Could you check a few things on this model? Use its own coordinates, in mm. Face numbers are marked on the shaded views. A direction names the side the tool comes from. Round coordinates to 2 decimals unless told otherwise and drop trailing zeros. Loops run counter-clockwise (first coordinate to the right, second up) from the corner with the lowest first, then second, coordinate; pieces in that order, holes last. Notation, with made-up numbers: M -2.5,30.5 L 52.5,30.5 A21 cw 52.5,37.5 Z; hole C 86.25,76 d8. An arc over 180 degrees is marked long. Answer in a Markdown table with one row per item.
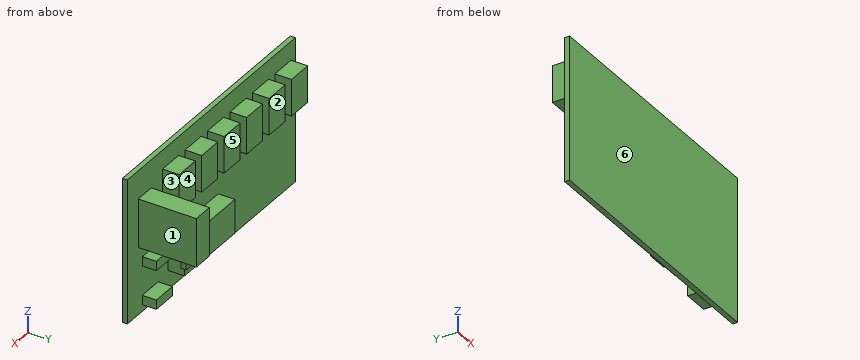
Autodesk Inventor part; units mm, degrees
ref_plane "YZ Plane" through (0, 0, 0) normal (1, 0, 0) x (0, 1, 0)
ref_plane "XZ Plane" through (0, 0, 0) normal (0, 1, 0) x (-1, 0, 0)
ref_plane "XY Plane" through (0, 0, 0) normal (0, 0, 1) x (1, 0, 0)
sketch "Sketch1" plane through (0, 0, 0) normal (0, 1, 0) x (-1, 0, 0)
  line L0 (-80, -43.475) -> (80, -43.475)
  line L1 (80, -43.475) -> (80, 43.475)
  line L2 (80, 43.475) -> (-80, 43.475)
  line L3 (-80, 43.475) -> (-80, -43.475)
  line L4 (-80, -43.475) -> (80, 43.475) construction
  line L5 (80, -43.475) -> (-80, 43.475) construction
  point P0 (0, 0)
  dimension "d0" = 160
  dimension "d1" = 86.95
extrude "Extrusion1" add sketch "Sketch1" along normal blind 3
sketch "Sketch2" plane through (0, 3, 0) normal (0, 1, 0) x (1, 0, 0)
  line L0 (-6.6, 31.775) -> (41.4, 31.775)
  line L1 (41.4, 31.775) -> (41.4, 11.375)
  line L2 (41.4, 11.375) -> (-6.6, 11.375)
  line L3 (-6.6, 11.375) -> (-6.6, 31.775)
  line L4 (80, -43.475) -> (80, 43.475)
  line L5 (-80, -43.475) -> (80, -43.475)
  line L6 (-75.9, -32.075) -> (-60.6, -32.075)
  line L7 (-60.6, -32.075) -> (-60.6, -9.975)
  line L8 (-60.6, -9.975) -> (-75.9, -9.975)
  line L9 (-75.9, -9.975) -> (-75.9, -32.075)
  line L10 (-80, 43.475) -> (-80, -43.475)
  line L11 (-54.5, -32.075) -> (-39.2, -32.075)
  line L12 (-39.2, -32.075) -> (-39.2, -9.975)
  line L13 (-39.2, -9.975) -> (-54.5, -9.975)
  line L14 (-54.5, -9.975) -> (-54.5, -32.075)
  line L15 (-33.1, -32.075) -> (-17.8, -32.075)
  line L16 (-17.8, -32.075) -> (-17.8, -9.975)
  line L17 (-17.8, -9.975) -> (-33.1, -9.975)
  line L18 (-33.1, -9.975) -> (-33.1, -32.075)
  line L19 (57.2, 2.825) -> (69.6, 2.825)
  line L20 (69.6, 2.825) -> (69.6, -26.475)
  line L21 (69.6, -26.475) -> (57.2, -26.475)
  line L22 (57.2, -26.475) -> (57.2, 2.825)
  line L23 (-11.7, -9.975) -> (-11.7, -32.075)
  line L24 (3.6, -9.975) -> (-11.7, -9.975)
  line L25 (3.6, -32.075) -> (3.6, -9.975)
  line L26 (-11.7, -32.075) -> (3.6, -32.075)
  line L27 (31.1, -9.975) -> (31.1, -32.075)
  line L28 (46.4, -9.975) -> (31.1, -9.975)
  line L29 (46.4, -32.075) -> (46.4, -9.975)
  line L30 (31.1, -32.075) -> (46.4, -32.075)
  line L31 (25, -9.975) -> (9.7, -9.975)
  line L32 (9.7, -32.075) -> (25, -32.075)
  line L33 (25, -32.075) -> (25, -9.975)
  line L34 (9.7, -9.975) -> (9.7, -32.075)
  line L35 (80, 43.475) -> (-80, 43.475)
  point P0 (0, 0)
  dimension "d6" = 48
  dimension "d7" = 20.4
  dimension "d26" = 15.3
  dimension "d27" = 22.1
  dimension "d29" = 4.1
  dimension "d30" = 15.3
  dimension "d32" = 15.3
  dimension "d36" = 12.4
  dimension "d37" = 29.3
  dimension "d38" = 15.3
  dimension "d42" = 15.3
  dimension "d44" = 15.3
  dimension "d46" = 6.1
  dimension "d47" = 6.1
  dimension "d48" = 6.1
  dimension "d49" = 6.1
  dimension "d50" = 6.1
  dimension "d51" = 11.4
  dimension "d52" = 10.4
  dimension "d53" = 17
  dimension "d54" = 73.4
  dimension "d55" = 11.7
extrude "Extrusion4" add sketch "Sketch2" along normal blind 10 contours L0 L1 L2 L3 | L9 L8 L7 L6 | L14 L13 L12 L11 | L18 L17 L16 L15 | L19 L20 L21 L22 | L24 L25 L26 L23 | L28 L29 L30 L27 | L33 L32 L34 L31
sketch "Sketch4" plane through (0, 13, 0) normal (0, 1, 0) x (1, 0, 0)
  line L0 (44.5244, 25.526) -> (38.2756, 25.526)
  line L1 (38.2756, 25.526) -> (38.2756, 17.624)
  line L2 (38.2756, 17.624) -> (44.5244, 17.624)
  line L3 (44.5244, 17.624) -> (44.5244, 25.526)
  line L4 (41.4, 11.375) -> (41.4, 31.775)
  line L5 (44.5244, 25.526) -> (38.2756, 17.624) construction
  line L6 (38.2756, 25.526) -> (44.5244, 17.624) construction
  point P0 (0, 0)
  point P1 (41.4, 21.575)
extrude "Extrusion5" add sketch "Sketch4" along normal blind 3
sketch "Sketch5" plane through (0, 3, 0) normal (0, 1, 0) x (1, 0, 0)
  line L0 (65.8, 16.025) -> (50.6, 16.025)
  line L1 (50.6, 16.025) -> (50.6, 10.425)
  line L2 (50.6, 10.425) -> (65.8, 10.425)
  line L3 (65.8, 10.425) -> (65.8, 16.025)
  line L4 (80, 43.475) -> (-80, 43.475)
  line L5 (80, -43.475) -> (80, 43.475)
  line L6 (65.8, 39.375) -> (50.6, 39.375)
  line L7 (50.6, 39.375) -> (50.6, 33.775)
  line L8 (50.6, 33.775) -> (65.8, 33.775)
  line L9 (65.8, 33.775) -> (65.8, 39.375)
  point P0 (0, 0)
  dimension "d60" = 15.2
  dimension "d61" = 5.6
  dimension "d62" = 27.45
  dimension "d63" = 14.2
  dimension "d64" = 15.2
  dimension "d65" = 5.6
  dimension "d66" = 4.1
extrude "Extrusion6" add sketch "Sketch5" along normal blind 8.5
sketch "Sketch6" plane through (0, 13, 0) normal (0, 1, 0) x (1, 0, 0)
  line L0 (57.2, -26.475) -> (69.6, -26.475)
  line L1 (69.6, -26.475) -> (57.2, -26.475)
  line L2 (57.2, -26.475) -> (57.2, 2.825)
  line L3 (57.2, 2.825) -> (69.6, 2.825)
  line L4 (69.6, 2.825) -> (69.6, -26.475)
  point P0 (0, 0)
extrude "Extrusion7" add sketch "Sketch6" along normal blind 25
properties part number "PCB"
1) If we mould it in two halves opening along X, with no side actions, what happens to the marked faces 1, 2 and 3? For each: released by +X, released by -X, zero draft, split by the parting line, or undercut.
Computed:
| item | result |
|---|---|
| face 1 | released by +X |
| face 2 | zero draft |
| face 3 | undercut |
2) Will these pins go through, and if not, where does the flat tip stop? P1, Ø5, axis at x = -43.5, y = 9.5, coming from the +Z side (3 decimals); P2, Ø14.5, axis at y = 24, z = 15.5, coming from the +X side; P3, Ø4.5, axis at y = 7, z = -13, coming from the -X side.
Computed:
| item | result |
|---|---|
| P1 | stops at z = 32.075 |
| P2 | stops at x = 69.6 |
| P3 | stops at x = -6.6 |
3) Which directions (+Z, -Z, +X, -X, +Y, -Y) give clear straight access to the entire face, cutting with the end or side of a thin tool? Please do the marked faces 4, 5 and 6.
Computed:
| item | result |
|---|---|
| face 4 | +Z, -X, +Y |
| face 5 | +Z, -Z, -X, +Y |
| face 6 | +Z, -Z, +X, -X, -Y |
4) I want a section at A-A, the plane z = -29. Please give me the cut outline in (x, y), plus the area to 3 significant figures.
Computed:
| item | result |
|---|---|
| outline | M -80,0 L 80,0 L 80,3 L 41.4,3 L 41.4,13 L -6.6,13 L -6.6,3 L -80,3 Z |
| area | 960 mm² |
5) I need wall thicknesses on line 1 (Y direction, x = -16, z = -7); line 2 (Y direction, x = 18, z = 23); line 3 (X direction, y = 17, z = 8). Which ranges of each line are inside material? Lowest first, please.
Computed:
| item | result |
|---|---|
| line 1 | y = 0 to 3 |
| line 2 | y = 0 to 13 |
| line 3 | x = 57.2 to 69.6 |
6) I want a section at D-D, the plane z = -14.5. Please give me the cut outline in (x, y).
Computed:
| item | result |
|---|---|
| outline | M -80,0 L 80,0 L 80,3 L 65.8,3 L 65.8,11.5 L 50.6,11.5 L 50.6,3 L 41.4,3 L 41.4,13 L -6.6,13 L -6.6,3 L -80,3 Z |
7) I want a section at B-B, the plane x = -23. Please give me the cut outline in (y, z) (3 decimals).
Computed:
| item | result |
|---|---|
| outline | M 0,-43.475 L 3,-43.475 L 3,9.975 L 13,9.975 L 13,32.075 L 3,32.075 L 3,43.475 L 0,43.475 Z |
8) I want a section at C-C, the plane y = 7. State how many separate pieces and enclosed holes the cut face has, plus the area to 3 significant figures.
Computed:
| item | result |
|---|---|
| separate pieces | 10 |
| enclosed holes | 0 |
| area | 3,540 mm² |
